Read the model definition and answer for the solid it produces. Units are mm, in the model's axes. A direction names the side the tool comes from. Coordinates: 2 decimals unless noted, no trailing zeros. Loops run counter-clockwise (first coordinate to the right, second up) from the corner with the lowest first, then second, coordinate; pieces in that order, holes last. Notation, with made-up numbers: (19, -5.75) -> (54, -5.75) arc R17 ccw to (54, 0.25) -> close; hole circle Ø1 at (51.5, 83.25). An arc over 180 degrees is marked (long way). Answer as a JSON object with one key per item and string values. Group by question number.
Q1. Each of these flat-tipped pins is pushed along its axis until it touches: P1, Ø2, axis at x = -63, z = 1, coming from the +Y side; P2, Ø1.2, axis at x = 2, z = 0.5, coming from the -Y side; P3, Ø12, axis at x = -139.5, y = 47.5, coming from the -Z side; P4, Ø2, axis at y = 69.5, z = 1, coming from the +X side. Where does it stop, or does it pass through?
Q2. Determine the mould class of faces 5 (the flat face through (-155, 68, 0)), 6 (the flat face through (-3, 9, 0)), 7 (the flat face through (-123.143, 53.604, 0.028)) for opening direction Y: released by +Y, released by -Y, zero draft, split by the parting line, or undercut.
Q3. The part is cut by section D-D on y = 29. Write down the section's boundary in (x, z), and give its area (3 significant figures).
Q4. The part is cut by section A-A on x = -4.5. Write down the section's boundary in (y, z), and give its area (3 significant figures).
Q5. Straight lines are drawn through the part: line 1 along X through (y, z) = (11, -0.05); line 2 along Y through (x, z) = (-71, 0.7); line 3 along X through (y, z) = (17, -1.25). For each, find the intervals that lie inside material, in ascending order. Write a range as [from, to].
Q6. For faces 1 (the flat face through (-29, 9, 0)), 2 (the flat face through (-125, 70, 0)), 3 (the flat face through (2, 43, 0)), 4 (the flat face through (2, 8, 0)), determine the directions among +Z, -Z, +X, -X, +Y, -Y from which every point of the face is accessible in a straight line to the end or side of a thin tool.
Q7. The part is cut by section B-B on x = -30.5. Write down the section's boundary in (y, z), and give its area (3 significant figures).
Q8. The part is cut by section C-C on z = 0.5. State how many separate pieces and enclosed holes the cut face has, and give its area (3 significant figures).
from build123d import *

# Parameters (mm, degrees)
BOSS_EXTRUDE1_DEPTH = 2
CUT_EXTRUDE1_REACH  = 186.662
SKETCH3_W           = 25
SKETCH3_H           = 4
CUT_EXTRUDE2_DEPTH  = 185.661853126
SKETCH4_W           = 4
SKETCH4_H           = 10
BOSS_EXTRUDE2_DEPTH = 4
CUT_EXTRUDE3_DEPTH  = 176.327288924


with BuildPart() as part:
    # Sketch1 → Boss-Extrude1 (new, symmetric)
    with BuildSketch(Plane.XY):
        Polygon((0, 4), (0, 72), (-170, 72), (-35, 19), (-35, 4), align=None)
    extrude(amount=BOSS_EXTRUDE1_DEPTH, both=True)

    # Sketch2 → Cut-Extrude1 (cut, up to next)
    with BuildSketch(Plane.XY.offset(2), mode=Mode.PRIVATE) as cut_extrude1_sk1:
        with BuildLine():
            Line((-3, 11), (-3, 7.5))
            ThreePointArc((-3, 7.5), (-4.5, 6), (-6, 7.5))
            Line((-6, 7.5), (-6, 11))
            ThreePointArc((-6, 11), (-4.5, 12.5), (-3, 11))
        make_face()
    cut_extrude1_tool1 = extrude(cut_extrude1_sk1.sketch, amount=-CUT_EXTRUDE1_REACH, mode=Mode.PRIVATE) & part.part
    # Sketch2 → Cut-Extrude1 (cut, up to next)
    with BuildSketch(Plane.XY.offset(2), mode=Mode.PRIVATE) as cut_extrude1_sk2:
        with BuildLine():
            Line((-32, 11), (-32, 7.5))
            ThreePointArc((-32, 7.5), (-30.5, 6), (-29, 7.5))
            Line((-29, 7.5), (-29, 11))
            ThreePointArc((-29, 11), (-30.5, 12.5), (-32, 11))
        make_face()
    cut_extrude1_tool2 = extrude(cut_extrude1_sk2.sketch, amount=-CUT_EXTRUDE1_REACH, mode=Mode.PRIVATE) & part.part
    add(cut_extrude1_tool1.solids().sort_by_distance((-4.5, 9.25, 2))[0], mode=Mode.SUBTRACT)
    add(cut_extrude1_tool2.solids().sort_by_distance((-30.5, 9.25, 2))[0], mode=Mode.SUBTRACT)

    # Sketch3 → Cut-Extrude2 (cut, through all)
    with BuildSketch(Plane.XY.offset(2)):
        with Locations((-62.5, 70)):
            Rectangle(SKETCH3_W, SKETCH3_H)
        with Locations((-12.5, 70)):
            Rectangle(SKETCH3_W, SKETCH3_H)
        with Locations((-112.5, 70)):
            Rectangle(SKETCH3_W, SKETCH3_H)
        with Locations((-162.5, 70)):
            Rectangle(SKETCH3_W, SKETCH3_H)
        with Locations((-212.5, 70)):
            Rectangle(SKETCH3_W, SKETCH3_H)
        with Locations((-262.5, 70)):
            Rectangle(SKETCH3_W, SKETCH3_H)
        with Locations((-312.5, 70)):
            Rectangle(SKETCH3_W, SKETCH3_H)
        with Locations((-362.5, 70)):
            Rectangle(SKETCH3_W, SKETCH3_H)
        with Locations((-412.5, 70)):
            Rectangle(SKETCH3_W, SKETCH3_H)
        with Locations((-462.5, 70)):
            Rectangle(SKETCH3_W, SKETCH3_H)
    extrude(amount=-CUT_EXTRUDE2_DEPTH, mode=Mode.SUBTRACT)

    # Sketch4 → Boss-Extrude2 (add)
    with BuildSketch(Plane(origin=(0, 0, 0), x_dir=(0, 0, -1), z_dir=(1, 0, 0))):
        with Locations((0, 63)):
            Rectangle(SKETCH4_W, SKETCH4_H)
        with Locations((0, 38)):
            Rectangle(SKETCH4_W, SKETCH4_H)
        with Locations((0, 13)):
            Rectangle(SKETCH4_W, SKETCH4_H)
    extrude(amount=BOSS_EXTRUDE2_DEPTH)

    # Sketch5 → Cut-Extrude3 (cut, through all)
    with BuildSketch(Plane.XY.offset(2)):
        with BuildLine():
            Line((-85.433962264, 38.8), (-46, 38.8))
            ThreePointArc((-46, 38.8), (-33, 25.8), (-46, 12.8))
            Line((-46, 12.8), (-85.433962264, 12.8))
            ThreePointArc((-85.433962264, 12.8), (-98.433962264, 25.8), (-85.433962264, 38.8))
        make_face()
    extrude(amount=-CUT_EXTRUDE3_DEPTH, mode=Mode.SUBTRACT)


solid = part.part
Final values:
{
 "1": {"P1": "stops at y = 68", "P2": "stops at y = 8", "P3": "passes through", "P4": "stops at x = -25"},
 "2": {"face 5": "released by +Y", "face 6": "undercut", "face 7": "released by -Y"},
 "3": {"outline": "(-33.4, -2) -> (0, -2) -> (0, 2) -> (-33.4, 2) -> close", "area": "134 mm2"},
 "4": {"outline": "(4, -2) -> (6, -2) -> (6, 2) -> (4, 2) -> close; (12.5, -2) -> (68, -2) -> (68, 2) -> (12.5, 2) -> close", "area": "230 mm2"},
 "5": {"line 1": "x = [-35, -32], [-29, -6], [-3, 4]", "line 2": "y = [38.8, 68]", "line 3": "x = [-35, 4]"},
 "6": {"face 1": "+Z, -Z", "face 2": "+Z, -Z, +Y", "face 3": "+Z, -Z, +X", "face 4": "+Z, -Z, +X, -Y"},
 "7": {"outline": "(4, -2) -> (6, -2) -> (6, 2) -> (4, 2) -> close; (12.5, -2) -> (72, -2) -> (72, 2) -> (12.5, 2) -> close", "area": "246 mm2"},
 "8": {"separate pieces": "1", "enclosed holes": "2", "area": "5,180 mm2"}
}
